Geometry: final body of the model. Coordinates: model frame, mm. Give positions to 0.01 mm unless a question says otherwise; leave off trailing zeros. Loops run counter-clockwise (first coordinate to the right, second up) from the corner with the lowest first, then second, coordinate; pieces in that order, holes last.
from build123d import *

# Parameters (mm, degrees)
SKETCH1_W            = 88.9
SKETCH1_H            = 431.8
BOSS_EXTRUDE1_DEPTH  = 5.8
M3_CLEARANCE_HOLE1_D = 3.4
SKETCH2_W            = 63.5
SKETCH2_H            = 368.3
CUT_EXTRUDE1_DEPTH   = 441.89464728
SKETCH3_W            = 8.5
SKETCH3_H            = 431.8
BOSS_EXTRUDE2_DEPTH  = 5.8
SKETCH7_R            = 0.79375
CUT_EXTRUDE2_DEPTH   = 443.68684191
SKETCH9_W            = 25.4
SKETCH9_H            = 95.25
BOSS_EXTRUDE3_DEPTH  = 5.8
SKETCH10_R           = 0.79375
CUT_EXTRUDE4_DEPTH   = 449.959597291
FILLET1_R            = 6.35


with BuildPart() as part:
    # Sketch1 → Boss-Extrude1 (new body)
    with BuildSketch(Plane(origin=(0, 0, 0), x_dir=(1, 0, 0), z_dir=(0, 1, 0))):
        with Locations((-44.45, -215.9)):
            Rectangle(SKETCH1_W, SKETCH1_H)
    extrude(amount=BOSS_EXTRUDE1_DEPTH)

    # M3 Clearance Hole1 (through all)
    with Locations(Plane(origin=(0, 5.8, 0), x_dir=(-1, 0, 0), z_dir=(0, 1, 0))):
        with Locations((82.55, 12.7), (6.35, 12.7), (6.35, 419.1), (82.55, 419.1), (82.55, 215.9), (6.35, 215.9)):
            Hole(M3_CLEARANCE_HOLE1_D / 2)

    # Sketch2 → Cut-Extrude1 (cut, through all)
    with BuildSketch(Plane(origin=(0, 5.8, 0), x_dir=(1, 0, 0), z_dir=(0, 1, 0))):
        with Locations((-44.45, -209.55)):
            Rectangle(SKETCH2_W, SKETCH2_H)
    extrude(amount=-CUT_EXTRUDE1_DEPTH, mode=Mode.SUBTRACT)

    # Sketch3 → Boss-Extrude2 (add, through all)
    with BuildSketch(Plane(origin=(0, 5.8, 0), x_dir=(-1, 0, 0), z_dir=(0, 1, 0))):
        with Locations((93.15, 215.9)):
            Rectangle(SKETCH3_W, SKETCH3_H)
    extrude(amount=-BOSS_EXTRUDE2_DEPTH)

    # Sketch7 → Cut-Extrude2 (cut, through all)
    with BuildSketch(Plane(origin=(0, 5.8, 0), x_dir=(1, 0, 0), z_dir=(0, 1, 0))):
        with Locations(Location((-44.45, -12.7, 0), (0, 0, 270))):
            Circle(SKETCH7_R)
        with Locations(Location((-82.55, -38.1, 0), (0, 0, 270))):
            Circle(SKETCH7_R)
        with Locations(Location((-6.35, -38.1, 0), (0, 0, 270))):
            Circle(SKETCH7_R)
        with Locations(Location((-6.35, -393.7, 0), (0, 0, 90))):
            Circle(SKETCH7_R)
        with Locations(Location((-82.55, -393.7, 0), (0, 0, 90))):
            Circle(SKETCH7_R)
        with Locations(Location((-44.45, -419.1, 0), (0, 0, 90))):
            Circle(SKETCH7_R)
    extrude(amount=-CUT_EXTRUDE2_DEPTH, mode=Mode.SUBTRACT)

    # Sketch9 → Boss-Extrude3 (add, through all)
    with BuildSketch(Plane(origin=(0, 5.8, 0), x_dir=(1, 0, 0), z_dir=(0, 1, 0))):
        with Locations((-110.1, -47.625)):
            Rectangle(SKETCH9_W, SKETCH9_H)
    extrude(amount=-BOSS_EXTRUDE3_DEPTH)

    # Sketch10 → Cut-Extrude4 (cut, through all)
    with BuildSketch(Plane(origin=(0, 5.8, 0), x_dir=(1, 0, 0), z_dir=(0, 1, 0))):
        with Locations(Location((-116.45, -88.9, 0), (0, 0, 270))):
            Circle(SKETCH10_R)
        with Locations(Location((-116.45, -6.35, 0), (0, 0, 270))):
            Circle(SKETCH10_R)
    extrude(amount=-CUT_EXTRUDE4_DEPTH, mode=Mode.SUBTRACT)

    # Fillet1
    fillet1_edges = [part.edges().sort_by_distance(p)[0] for p in [
        (0, 2.9, 431.8),
        (-97.4, 2.9, 431.8),
        (-122.8, 2.9, 95.25),
        (0, 2.9, 0),
        (-122.8, 2.9, 0),
    ]]
    fillet(fillet1_edges, radius=FILLET1_R)


solid = part.part
Item 1: Section query C-C on y = 1.35. Give the number of separate pieces and of enclosed holes in the cut face, plus the area to 3 significant figures.
Values follow:
separate pieces: 1
enclosed holes: 15
area: 21,000 mm2
Item 2: Ray query, probe 1 along Z at (x, y) = (-82.55, 2.55); probe 2 along X at (y, z) = (3, 419.1); probe 3 along Z at (x, y) = (-116.5, 0.9). Return the intervals inside material, ascending.
Values follow:
probe 1: z = 0 to 11, 14.4 to 37.31, 38.89 to 214.2, 217.6 to 392.91, 394.49 to 417.4, 420.8 to 431.8
probe 2: x = -97.4 to -84.25, -80.85 to -45.24, -43.66 to -8.05, -4.65 to 0
probe 3: z = 0 to 5.56, 7.14 to 88.11, 89.69 to 95.25
Item 3: Section query A-A on z = 200. Return loops of the section in (x, y), plus the area to 3 significant figures.
Values follow:
outline: (-97.4, 0) - (-76.2, 0) - (-76.2, 5.8) - (-97.4, 5.8) - close; (-12.7, 0) - (0, 0) - (0, 5.8) - (-12.7, 5.8) - close
area: 197 mm2
Item 4: Section query B-B on x = -23.5. Return loops of the section in (y, z), plus the area to 3 significant figures.
Values follow:
outline: (0, 0) - (5.8, 0) - (5.8, 25.4) - (0, 25.4) - close; (0, 393.7) - (5.8, 393.7) - (5.8, 431.8) - (0, 431.8) - close
area: 368 mm2
Item 5: Pin query (flat end, axial travel): pin 1 (3 mm diameter, centred on y = 2.5, z = 152.5, fed in from -X). Return the tip coordinate at first contact, or that it passes through.
Values follow:
pin 1: stops at x = -97.4
